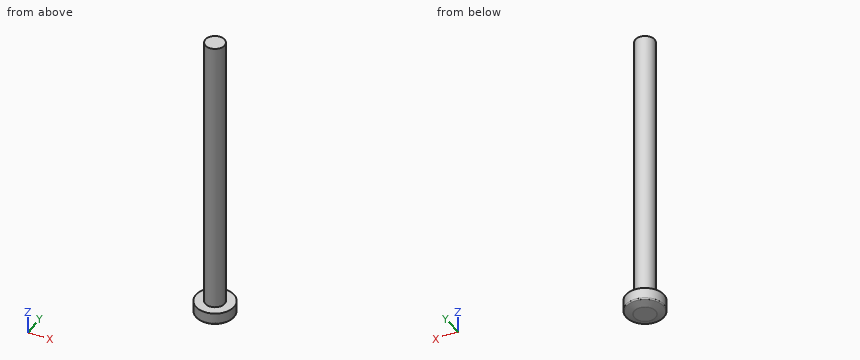
Autodesk Inventor part; units mm, degrees
ref_plane "YZ Plane" through (0, 0, 0) normal (1, 0, 0) x (0, 1, 0)
ref_plane "XZ Plane" through (0, 0, 0) normal (0, 1, 0) x (-1, 0, 0)
ref_plane "XY Plane" through (0, 0, 0) normal (0, 0, 1) x (1, 0, 0)
sketch "Sketch1" plane through (0, 0, 0) normal (0, 0, 1) x (1, 0, 0)
  circle A0 centre (0, 0) radius 3.375
  dimension "d0" = 6.75
extrude "Extrusion1" add sketch "Sketch1" along normal blind 2.6
sketch "Sketch2" plane through (0, 0, 2.6) normal (0, 0, 1) x (1, 0, 0)
  circle A0 centre (0, 0) radius 1.7
  dimension "d3" = 3.4
extrude "Extrusion2" add sketch "Sketch2" along normal blind 50
thread "Thread1"
chamfer "Chamfer1" distance 1.5 angle 20 1 edges at (-3.375, 0, 0) measured on face at (1.1885, -0.5228, 0)
fillet "Fillet1" radius 0.25 2 edges at (-3.375, 0, 0.546) (-1.875, 0, 0)
properties part number "6-32_Bolt"
The model under review builds one solid part; all positions refer to its coordinate system, in mm. Give positions to 0.01 mm unless a question says otherwise; leave off trailing zeros. Order: outer loops, then holes, each group sorted by start corner. A loop starts at its lowest first (then second) coordinate and runs counter-clockwise, first axis right, second up. Notation, with made-up numbers: (-28, -38.5) - (-15, -38.5) arc R19 ccw to (-15, -23.5) - close; hole circle Ø6 at (43.25, -13.75). An arc over 180 degrees is marked (long way). Use CSV: the item, a comma, the result in double quotes. Start each with the question number.
Q1. To check wall thickness, follow line 1 along Y through (x, z) = (0, 8.5); line 2 along Z through (x, y) = (0.5, -1.75); line 3 along X through (y, z) = (-0.75, 35). State the ranges of each line that lie inside material, in increasing order. Write a range as [from, to].
Q2. We need section A-A, the plane z = 23. Write out the cut boundary in (x, y).
Q3. Clearance check with flat-ended pins moving along their axes: pin 1 Ø2 at (y, z) = (-1.5, 27.5) entering from +X; pin 2 Ø1 at (y, z) = (0, 19.5) entering from +X. State where each tip first meets the part, or that it passes through.
Outcome:
1,line 1,"y = [-1.7, 1.7]"
1,line 2,"z = [0, 2.6]"
1,line 3,"x = [-1.53, 1.53]"
2,outline,"circle Ø3.4 at (0, 0)"
3,pin 1,"stops at x = 1.62"
3,pin 2,"stops at x = 1.7"
